The figure shows three views and two pictorial views of one solid part (mm, origin at its lowest corner). Answer the questions. A direction names the side the tool comes from. Coordinates: 2 decimals unless noted, no trailing zeros. Write each loop counter-clockwise with the first axis right and the second up, starting at its lowest first coordinate (ties: lowest second). Pieces come first, ordered by that corner, then holes.
Item 1: A tool of negligible diameter and unlimited length cuts with its end or side. For the marked faces 1 and 2, from which of +Z, -Z, +X, -X, +Y, -Y can it reach the whole face along a straight path? Write none if from no direction.
Item 2: Section B-B (y = 34) is taken. Give the vertices of the cut face in (x, z).
Item 3: Section C-C (x = 12.5) is taken. Give the vertices of the cut face in (y, z), then the cut area to 3 significant figures.
Item 4: Straight lines are drawn through the part: probe 1 along Z at (x, y) = (25, 38); probe 2 along Z at (x, y) = (30.5, 31); probe 3 along X at (y, z) = (2.5, 8). For each, find the intervals that lie inside material, in ascending order.
Item 5: Section D-D (z = 42) is taken. Give the vertices of the cut face in (x, y) (1 decimal), then the cut area to 3 significant figures.
Item 6: Each of these flat-tipped pins is pushed along its axis until it touches: P1, Ø6, axis at x = 29, z = 51.5, coming from the -Y side (1 decimal); P2, Ø1.5, axis at x = 26.5, y = 48, coming from the +Z side; P3, Ø2.5, axis at x = 4.5, y = 27, coming from the +Z side. Where does it stop, or does it pass through?
Item 7: Section A-A (z = 24) is taken. Give the vertices of the cut face in (x, y).
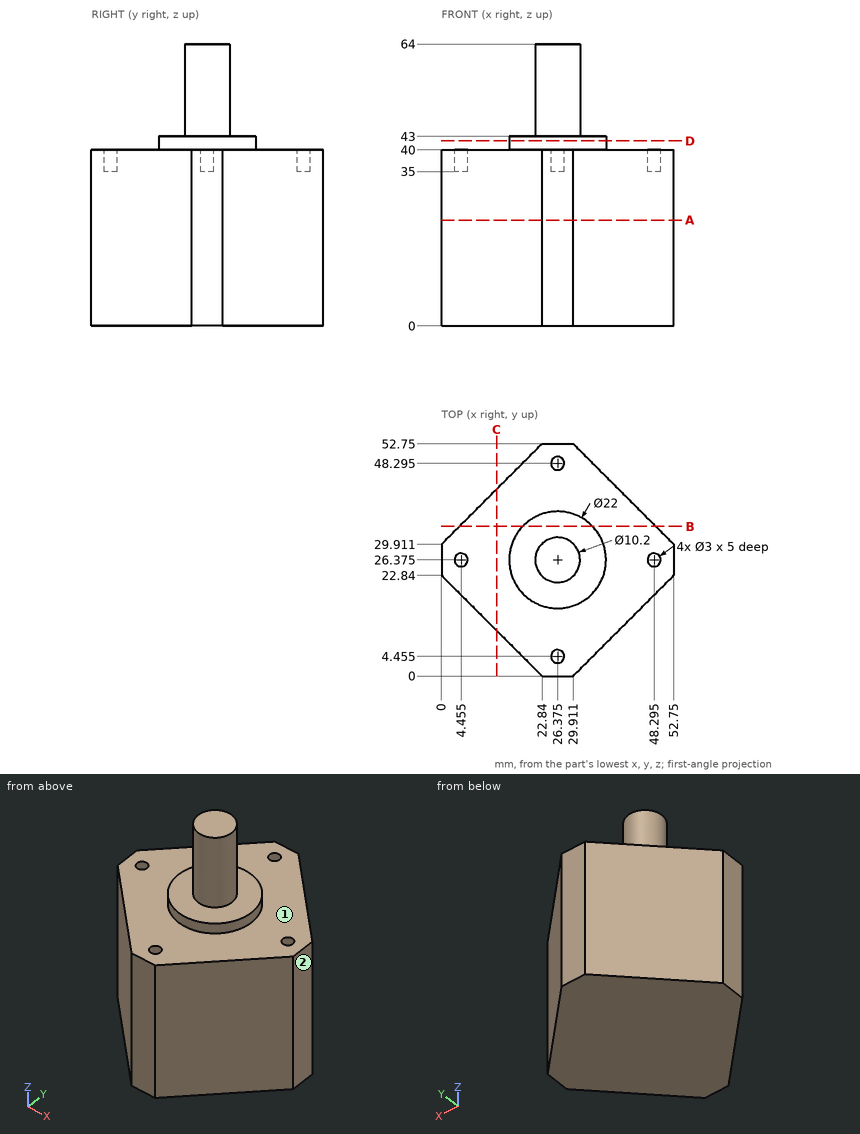
Established:
1. face 1: +Z
1. face 2: +Z, -Z, +X, +Y, -Y
2. outline: (4.09, 0) - (48.66, 0) - (48.66, 40) - (34.3, 40) - (34.3, 43) - (18.45, 43) - (18.45, 40) - (4.09, 40) - close
3. outline: (10.34, 0) - (42.41, 0) - (42.41, 40) - (10.34, 40) - close
3. area: 1,280 mm2
4. probe 1: z = 0 to 40
4. probe 2: z = 0 to 43
4. probe 3: x = 20.34 to 32.41
5. outline: circle Ø22 at (26.4, 26.4)
5. area: 380 mm2
6. P1: stops at y = 21.3
6. P2: stops at z = 35
6. P3: stops at z = 40
7. outline: (0, 22.84) - (22.84, 0) - (29.91, 0) - (52.75, 22.84) - (52.75, 29.91) - (29.91, 52.75) - (22.84, 52.75) - (0, 29.91) - close
